Could you check a few things on this model? Use its own coordinates, in mm. A direction names the side the tool comes from. Coordinates: 2 decimals unless noted, no trailing zeros. Write each loop counter-clockwise with the first axis right and the second up, starting at its lowest first coordinate (ties: lowest second). Pieces come first, ordered by that corner, then holes. Notation, with made-up numbers: M 79,-17.5 L 120,-17.5 A24 cw 120,13.5 Z; hole C 76.5,19 d1. An arc over 180 degrees is marked long. Write item = value, one per line.
```python
from build123d import *

# Parameters (mm, degrees)
F0_W      = 10
F0_H      = 70
F1_DEPTH  = 145
F2_DEPTH  = 5
F3_W      = 8.287649136
F3_H      = 57.6572036371
F4_DEPTH  = 140
F5_W      = 2.6011180505
F5_H      = 57.6572036371
F6_DEPTH  = 120
F8_DEPTH  = 10
F10_DEPTH = 7


with BuildPart() as f1:
    # F0 (on Top) → F1 (new body)
    with BuildSketch(Plane.XY):
        with Locations((-5.0640162081, 34.8435932503)):
            Rectangle(F0_W, F0_H)
    extrude(amount=F1_DEPTH)

    # F2 (add): a face of the model
    f2_faces = [f1.faces().sort_by_distance(p)[0] for p in [
        (-0.0640162081, 34.8435932503, 72.5),
    ]]
    extrude(f2_faces, amount=F2_DEPTH)

    # F3 (on face) → F4 (cut)
    with BuildSketch(Plane.XY.offset(145)):
        with Locations((-1.8089588266, 34.3119842)):
            Rectangle(F3_W, F3_H)
    extrude(amount=-F4_DEPTH, mode=Mode.SUBTRACT)

    # F5 (on face) → F6 (cut)
    with BuildSketch(Plane.XY.offset(145)):
        with Locations((3.6354247667, 34.3119842)):
            Rectangle(F5_W, F5_H)
    extrude(amount=-F6_DEPTH, mode=Mode.SUBTRACT)

    # F7 (on face) → F8 (join)
    with BuildSketch(Plane(origin=(0, 5.4833823815, 0), x_dir=(-1, 0, 0), z_dir=(0, 1, 0))):
        Polygon((0.5083998013, 25), (0.5083998013, 145), (-4.9359837919, 145), (-4.9359837919, 25), (-2.3348657414, 25), align=None)
    extrude(amount=F8_DEPTH)

    # F9 (on face) → F10 (join)
    with BuildSketch(Plane.XZ.offset(-63.1405860186)):
        Polygon((4.9359837919, 145), (-0.5083998013, 145), (-0.5083998013, 25), (2.3348657414, 25), (4.9359837919, 25), align=None)
    extrude(amount=F10_DEPTH)


solid = f1.part
```
Item 1: Imagine slicing it at A-A (z = 18.5). Write out the boundary of the cut face in (x, y), and give its area (3 significant figures).
Numbers:
outline = M -10.06,-0.16 L 4.94,-0.16 L 4.94,69.84 L -10.06,69.84 Z; hole M -5.95,5.48 L 2.33,5.48 L 2.33,63.14 L -5.95,63.14 Z
area = 572 mm²
Item 2: If I drill on line 1 along X through (y, z) = (7, 27.5); line 2 along Y through (x, z) = (3, 54); line 3 along Y through (x, z) = (-3.5, 77.5), over which ranges is the centre line in solid material (lowest first)?
Numbers:
line_1 = -10.06 to -5.95, -0.51 to 4.94
line_2 = -0.16 to 15.48, 56.14 to 69.84
line_3 = -0.16 to 5.48, 63.14 to 69.84
Item 3: For faces 4 (the face through (4.936, 12, 55)), 5 (the face through (-3, -0.156, 71)), 6 (the face through (1, 10, 25)), 7 (the face through (-0.508, 60, 86)), 8 (the face through (4, 36, 25)), which set-ups out of +Z, -Z, +X, -X, +Y, -Y let a thin tool reach every point of the face, with its end or its side?
Numbers:
face_4 = +Z, -Z, +X, +Y, -Y
face_5 = +Z, -Z, +X, -X, -Y
face_6 = none
face_7 = +Z
face_8 = +Z, +X
Item 4: I'm going to push flat-ended pins straight in: P1, Ø3, axis at x = 4, y = 34.5, coming from the +Z side; P2, Ø1.5, axis at y = 23, z = 96.5, coming from the +X side; P3, Ø4, axis at x = -1, y = 24, coming from the +Z side. Where does each tip first touch, or does it pass through?
Numbers:
P1 = 25
P2 = -5.95
P3 = 5
Item 5: If we mould it in two halves opening along Z, with no side actions, what happens to faces 1 (the face through (1, 60, 25)), 2 (the face through (2, 56.141, 86)), 3 (the face through (-3, 34, 0))? For each: pulls with the +Z half, pulls with the -Z half, needs draft (parallel to the pull), parting line crosses it, or undercut.
Numbers:
face_1 = undercut
face_2 = needs draft
face_3 = pulls with the -Z half
Item 6: Imagine slicing it at C-C (y = 17). Write out the boundary of the cut face in (x, z).
Numbers:
outline = M -10.06,0 L 4.94,0 L 4.94,25 L 2.33,25 L 2.33,5 L -5.95,5 L -5.95,145 L -10.06,145 Z
Item 7: Imagine slicing it at B-B (x = -4.5). Write out the boundary of the cut face in (y, z), and give its area (3 significant figures).
Numbers:
outline = M -0.16,0 L 69.84,0 L 69.84,145 L 63.14,145 L 63.14,5 L 5.48,5 L 5.48,145 L -0.16,145 Z
area = 2,080 mm²
Item 8: Imagine slicing it at D-D (z = 117.5). Write out the boundary of the cut face in (x, y).
Numbers:
outline = M -10.06,-0.16 L 4.94,-0.16 L 4.94,15.48 L -0.51,15.48 L -0.51,5.48 L -5.95,5.48 L -5.95,63.14 L -0.51,63.14 L -0.51,56.14 L 4.94,56.14 L 4.94,69.84 L -10.06,69.84 Z
